```python
from build123d import *

# Parameters (mm, degrees)
F1_DEPTH = 63.5
F0_W     = 25.4
F0_H     = 19.05
F2_DEPTH = 25.4
F3_DEPTH = 7.9375
F5_R     = 6.35


with BuildPart() as f1:
    # F0 (on Front) → F1 (new body, symmetric)
    with BuildSketch(Plane.XZ):
        Polygon((-41.275, 9.525), (-41.275, -9.525), (41.275, -9.525), (41.275, 9.525), (22.225, 9.525), align=None)
    extrude(amount=F1_DEPTH, both=True)

    # F0 (on Front) → F2 (join, symmetric)
    with BuildSketch(Plane.XZ):
        with BuildLine():
            Line((22.225, 9.525), (41.275, 9.525))
            Line((41.275, 9.525), (41.275, 30.8000269385))
            ThreePointArc((41.275, 30.8000269385), (45.9246798487, 42.0253470898), (57.15, 46.6750269385))
            Line((57.15, 46.6750269385), (62.8952502342, 46.6750269385))
            Line((62.8952502342, 46.6750269385), (62.8952502342, 65.7250269385))
            Line((62.8952502342, 65.7250269385), (57.15, 65.7250269385))
            ThreePointArc((57.15, 65.7250269385), (32.4542956671, 55.4957312714), (22.225, 30.8000269385))
            Line((22.225, 30.8000269385), (22.225, 9.525))
        make_face()
        with Locations((75.5952502342, 56.2000269385)):
            Rectangle(F0_W, F0_H)
    extrude(amount=F2_DEPTH, both=True)

    # F0 (on Front) → F3 (join, symmetric)
    with BuildSketch(Plane.XZ):
        with BuildLine():
            add(Edge.make_bspline(
                [(-41.275, 9.525), (-19.8715052223, 41.4688585122), (21.5158074969, 68.07404407), (57.15, 65.7250269385)],
                knots=[0, 0, 0, 0, 113.3398590651, 113.3398590651, 113.3398590651, 113.3398590651], degree=3))
            Line((-41.275, 9.525), (22.225, 9.525))
            Line((22.225, 9.525), (22.225, 30.8000269385))
            ThreePointArc((22.225, 30.8000269385), (32.4542956671, 55.4957312714), (57.15, 65.7250269385))
        make_face()
    extrude(amount=F3_DEPTH, both=True)

    # F0 (on Front) → F4 (revolve)
    with BuildSketch(Plane.XZ):
        Polygon((88.2952502342, 67.1590872239), (88.2952502342, 65.7250269385), (88.2952502342, 46.6750269385), (88.2952502342, 38.5840872239), (113.6952502342, 38.5840872239), (113.6952502342, 67.1590872239), align=None)
    revolve(axis=Axis((88.2952502342, 0, 52.8715872239), (0, 0, 1)))

    # F5
    f5_edges = [f1.edges().sort_by_distance(p)[0] for p in [
        (41.275, -63.5, 0),
        (-41.275, -63.5, 0),
        (41.275, 63.5, 0),
    ]]
    fillet(f5_edges, radius=F5_R)


solid = f1.part
```
The listing builds one solid part. Answer for the finished solid, in the listing's coordinates (mm). A direction names the side the tool comes from. Round coordinates to 2 decimals unless told otherwise and drop trailing zeros. Loops run counter-clockwise (first coordinate to the right, second up) from the corner with the lowest first, then second, coordinate; pieces in that order, holes last. Notation, with made-up numbers: (67.5, 27) - (94.5, 27) arc R27 cw to (94.5, 49) - close; hole circle Ø10 at (50.25, 6.25). An arc over 180 degrees is marked (long way). Return JSON: item names as keys, results as strings. Group by question number.
1. Which of the six approach directions +Z, -Z, +X, -X, +Y, -Y give full straight-line access (tool end or side, diameter ignored) to faces 5 (the flat face through (47, 25.4, 44)), 6 (the flat face through (22.225, 17, 20)), 7 (the flat face through (41.275, -1, 6)), 8 (the flat face through (47, -25.4, 44)), 9 (the flat face through (-2, -7.938, 33))?
2. The part is cut by section A-A on z = 1. Determine the outline of the cut face in (x, y) (3 decimals), then the cut area to 3 significant figures.
3. The part is cut by section B-B on y = -12.5. Determine the outline of the cut face in (x, z) (3 decimals).
4. Each of these flat-tipped pins is pushed along its axis until it touches: P1, Ø1, axis at y = -20.5, z = 16.5, coming from the +X side (3 decimals); P2, Ø8.5, axis at y = -12.5, z = 21.5, coming from the -X side (3 decimals); P3, Ø8, axis at x = 35.5, z = 36.5, coming from the +Y side. Where does it stop, or does it pass through?
5. Consider probe 1 along X at (y, z) = (-20, 25) (3 decimals); probe 2 along Y at (x, z) = (85.5, 52.5); probe 3 along X at (y, z) = (-38, 8) (3 decimals). Determine where each line is inside the solid, lowest interval first.
6. The part is cut by section C-C on y = -49. Determine the outline of the cut face in (x, z) (3 decimals).
7. The mould has two halves that part along X. Classify faces 1 (the flat face through (-2, 7.938, 33)), 2 (the cylindrical face through (45.8, -0.4, 41.9)), 3 (the flat face through (62, 0, 65.725)), 4 (the flat face through (22.225, -17, 20)): pulls with the +X half, pulls with the -X half, needs draft (parallel to the pull), parting line crosses it, or undercut.
Resolved:
{
 "1": {"face 5": "+Z, +X, -X, +Y", "face 6": "+Z, -X, +Y", "face 7": "-Z, +X, +Y, -Y", "face 8": "+Z, +X, -X, -Y", "face 9": "+Z, -X, -Y"},
 "2": {"outline": "(-41.275, -57.15) arc R6.35 ccw to (-34.925, -63.5) - (34.925, -63.5) arc R6.35 ccw to (41.275, -57.15) - (41.275, 57.15) arc R6.35 ccw to (34.925, 63.5) - (-41.275, 63.5) - close", "area": "10,500 mm²"},
 "3": {"outline": "(-41.275, -9.525) - (41.275, -9.525) - (41.275, 30.8) arc R15.875 cw to (57.15, 46.675) - (66.184, 46.675) - (66.184, 38.584) - (110.407, 38.584) - (110.407, 67.159) - (66.184, 67.159) - (66.184, 65.725) - (57.15, 65.725) arc R34.925 ccw to (22.225, 30.8) - (22.225, 9.525) - (-41.275, 9.525) - close"},
 "4": {"P1": "stops at x = 41.275", "P2": "stops at x = 22.225", "P3": "stops at y = 25.4"},
 "5": {"probe 1": "x = 22.225 to 41.275", "probe 2": "y = -25.4 to 25.4", "probe 3": "x = -41.275 to 41.275"},
 "6": {"outline": "(-41.275, -9.525) - (41.275, -9.525) - (41.275, 9.525) - (-41.275, 9.525) - close"},
 "7": {"face 1": "needs draft", "face 2": "undercut", "face 3": "undercut", "face 4": "pulls with the -X half"}
}
